from build123d import *

# Parameters (mm, degrees)
SKETCH1_R           = 9.525
BOSS_EXTRUDE1_DEPTH = 38.1
SKETCH2_R           = 3.175
BOSS_EXTRUDE2_DEPTH = 101.6
SKETCH3_R           = 3.175
BOSS_EXTRUDE3_DEPTH = 101.6


with BuildPart() as part:
    # Sketch1 → Boss-Extrude1 (new, symmetric)
    with BuildSketch(Plane.XY):
        with Locations(Location((0, 0, 0), (0, 0, 180))):
            Circle(SKETCH1_R)
    extrude(amount=BOSS_EXTRUDE1_DEPTH, both=True)

    # Sketch2 → Boss-Extrude2 (add)
    with BuildSketch(Plane(origin=(0, 0, 0), x_dir=(0, 0, -1), z_dir=(1, 0, 0))):
        with Locations((-31.75, 0)):
            Circle(SKETCH2_R)
        with Locations((31.75, 0)):
            Circle(SKETCH2_R)
    extrude(amount=BOSS_EXTRUDE2_DEPTH)

    # Sketch3 → Boss-Extrude3 (add)
    with BuildSketch(Plane(origin=(0, 0, 0), x_dir=(1, 0, 0), z_dir=(0, 1, 0))):
        with Locations(Location((0, 31.75, 0), (0, 0, 90))):
            Circle(SKETCH3_R)
        with Locations(Location((0, -31.75, 0), (0, 0, 90))):
            Circle(SKETCH3_R)
    extrude(amount=BOSS_EXTRUDE3_DEPTH)


solid = part.part
Read the model definition and answer for the solid it produces. Units are mm, in the model's axes. A direction names the side the tool comes from. Round coordinates to 2 decimals unless told otherwise and drop trailing zeros. Write each loop counter-clockwise with the first axis right and the second up, starting at its lowest first coordinate (ties: lowest second). Pieces come first, ordered by that corner, then holes. Notation, with made-up numbers: (11, 40.25) - (40, 40.25) arc R23 cw to (40, 48.25) - close; hole circle Ø9 at (53.5, 35). An arc over 180 degrees is marked (long way). One line per question, with ' | ' between items. Start each with the question number.
1. For faces 1 (the face through (-0.14, 54.63, -28.58)), 2 (the face through (-9.085, -2.861, 0.533)), 3 (the face through (54.64, 0.14, -28.58)), determine the directions among +Z, -Z, +X, -X, +Y, -Y from which every point of the face is accessible in a straight line to the end or side of a thin tool.
2. Section D-D (y = 80) is taken. Determine the outline of the cut face in (x, z) (3 decimals).
3. Find the intervals of material crossed by probe 1 along Z at (x, y) = (13, -2); probe 2 along Y at (x, z) = (-0.5, 16); probe 3 along X at (y, z) = (74.5, 31), in increasing order. Write a range as [from, to].
4. Each of these flat-tipped pins is pushed along its axis until it touches: pin 1 (10 mm diameter, centred on x = 54.5, z = -24, fed in from -Y); pin 2 (6 mm diameter, centred on x = 2, z = -15.5, fed in from +Y) (3 decimals); pin 3 (1 mm diameter, centred on x = 5.5, z = -25.5, fed in from -Y). Where does it stop, or does it pass through?
5. Section A-A (y = 0) is taken. Determine the outline of the cut face in (x, z) (3 decimals), and give its area (3 significant figures).
6. For a pull along Z with two mould halves and no side action, classify faces 4 (the face through (54.64, 0.14, 34.92)), 5 (the face through (101.6, 0, -32)), 6 (the face through (0, 0, -38.1)) as +Z half, -Z half, draft (parallel to the pull), parting line (faces both ways), or undercut.
7. Section B-B (z = -31.75) is taken. Determine the outline of the cut face in (x, y) (3 decimals), and give its area (3 significant figures).
Filled in:
1) face 1: +Y | face 2: none | face 3: +X
2) outline: circle Ø6.35 at (0, -31.75); circle Ø6.35 at (0, 31.75)
3) probe 1: [-34.22, -29.28], [29.28, 34.22] | probe 2: [-9.51, 9.51] | probe 3: [-3.09, 3.09]
4) pin 1: y = -1.59 | pin 2: y = 9.525 | pin 3: y = -8.11
5) outline: (-9.525, -38.1) - (9.525, -38.1) - (9.525, -34.925) - (101.6, -34.925) - (101.6, -28.575) - (9.525, -28.575) - (9.525, 28.575) - (101.6, 28.575) - (101.6, 34.925) - (9.525, 34.925) - (9.525, 38.1) - (-9.525, 38.1) - close | area: 2,620 mm²
6) face 4: undercut | face 5: draft | face 6: -Z half
7) outline: (-3.175, 8.98) arc R9.525 ccw (long way) to (8.98, -3.175) - (101.6, -3.175) - (101.6, 3.175) - (8.98, 3.175) arc R9.525 ccw to (3.175, 8.98) - (3.175, 101.6) - (-3.175, 101.6) - close | area: 1,460 mm²
